from build123d import *

# Parameters (mm, degrees)
F0_W     = 10
F0_H     = 10
F1_DEPTH = 18
F2_R     = 1.5
F3_DEPTH = 7.5
F4_R     = 1.5
F5_DEPTH = 12.5


# Not quite as in the source:
# - a pattern or mirror of a feature is missing from the dataset's text; its kind, count and spacing are read off the source's solid


with BuildPart() as f1:
    # F0 (on Top) → F1 (new body, symmetric)
    with BuildSketch(Plane.XY):
        Rectangle(F0_W, F0_H)
    extrude(amount=F1_DEPTH, both=True)

    # F2 (on face) → F3 (cut)
    with BuildSketch(Plane.XY.offset(18)):
        Circle(F2_R)
    f3 = extrude(amount=-F3_DEPTH, mode=Mode.SUBTRACT)

    # F3_copies: F3 across plane
    add(f3.mirror(Plane(origin=(0, 0, 0), x_dir=(-1, 0, 0), z_dir=(0, 0, -1))), mode=Mode.SUBTRACT)

    # F4 (on Front) → F5 (cut, symmetric)
    with BuildSketch(Plane.XZ):
        with Locations((0, 8)):
            Circle(F4_R)
    f5 = extrude(amount=F5_DEPTH, both=True, mode=Mode.SUBTRACT)

    # F5_copies: F5 across plane
    add(f5.mirror(Plane(origin=(0, 0, 0), x_dir=(-1, 0, 0), z_dir=(0, 0, -1))), mode=Mode.SUBTRACT)


solid = f1.part
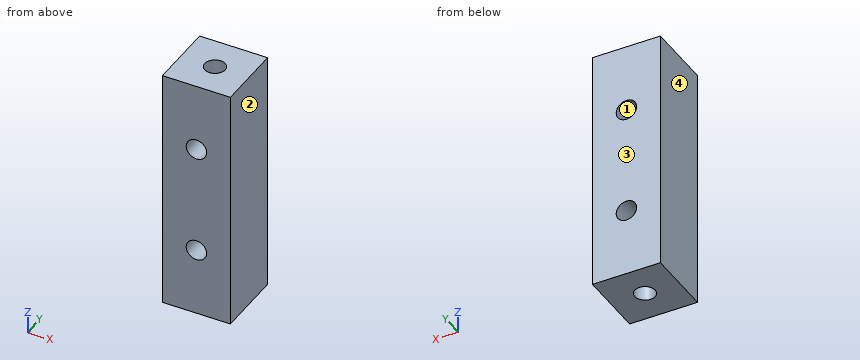
Check sheet for the modelled part. Datum: model origin and axes. Units: mm. Face numbers are marked on the shaded views. Round coordinates to 2 decimals unless told otherwise and drop trailing zeros. Order: outer loops, then holes, each group sorted by start corner. A loop starts at its lowest first (then second) coordinate and runs counter-clockwise, first axis right, second up.
(1) Go/stop test with flat-tipped pins: P1, Ø1.5, axis at x = -0.5, y = 0.5, coming from the +Z side; P2, Ø0.9, axis at x = 0, y = 0, coming from the -Z side. Record where each tip stops, or that it passes through.
(2) Cross-section at A-A, the plane x = 0. Enter the section's corners in (y, z).
(3) Cross-section at D-D, the plane z = -12. Enter the section's corners in (x, y).
(4) Draft check along X on the marked faces 1, 2, 3 and 4. Enter one of: pulls with the +X half, pulls with the -X half, needs draft (parallel to the pull), parting line crosses it, or undercut.
(5) Scan lines: probe 1 along Z at (x, y) = (0, 0.5); probe 2 along Y at (x, z) = (0, 12.75); probe 3 along Z at (x, y) = (-1, -2.75). Record each from-to range of solid material in increasing order.
(6) Cross-section at B-B, the plane z = -8. Enter the section's corners in (x, y).
(7) Cross-section at C-C, the plane y = 0. Enter the section's corners in (x, z), and give its area (3 significant figures).
Check sheet entries:
1. P1: stops at z = 10.5
1. P2: stops at z = -10.5
2. outline: (-5, -18) - (-1.5, -18) - (-1.5, -10.5) - (1.5, -10.5) - (1.5, -18) - (5, -18) - (5, -9.5) - (-5, -9.5) - close; (-5, -6.5) - (5, -6.5) - (5, 6.5) - (-5, 6.5) - close; (-5, 9.5) - (5, 9.5) - (5, 18) - (1.5, 18) - (1.5, 10.5) - (-1.5, 10.5) - (-1.5, 18) - (-5, 18) - close
3. outline: (-5, -5) - (5, -5) - (5, 5) - (-5, 5) - close; hole circle Ø3 at (0, 0)
4. face 1: undercut
4. face 2: pulls with the +X half
4. face 3: needs draft
4. face 4: pulls with the -X half
5. probe 1: z = -10.5 to -9.5, -6.5 to 6.5, 9.5 to 10.5
5. probe 2: y = -5 to -1.5, 1.5 to 5
5. probe 3: z = -18 to -9.12, -6.88 to 6.88, 9.12 to 18
6. outline: (-5, -5) - (-1.5, -5) - (-1.5, 5) - (-5, 5) - close; (1.5, -5) - (5, -5) - (5, 5) - (1.5, 5) - close
7. outline: (-5, -18) - (-1.5, -18) - (-1.5, -10.5) - (1.5, -10.5) - (1.5, -18) - (5, -18) - (5, 18) - (1.5, 18) - (1.5, 10.5) - (-1.5, 10.5) - (-1.5, 18) - (-5, 18) - close; hole circle Ø3 at (0, -8); hole circle Ø3 at (0, 8)
7. area: 301 mm2
